```python
from build123d import *

# Parameters (mm, degrees)
BOSS_EXTRUDE9_DEPTH      = 12.7
SKETCH2_R                = 5.08
CUT_EXTRUDE1_DEPTH       = 1
CUT_EXTRUDE1_DEPTH_BACK  = 13.7
SKETCH4_R                = 5.08
CUT_EXTRUDE3_DEPTH       = 13.7
SKETCH6_W                = 63.5
SKETCH6_H                = 63.5
CUT_EXTRUDE10_DEPTH      = 8.382
SKETCH8_R                = 1.2954
CUT_EXTRUDE13_DEPTH      = 5.318
SKETCH20_R               = 1.045475937
SKETCH20_R_2             = 1.05
SKETCH20_R_3             = 1.053113333
SKETCH20_R_4             = 1.049702702
SKETCH20_R_5             = 1.060351353
SKETCH20_R_6             = 1.041366857
CUT_EXTRUDE14_DEPTH      = 5.318
SKETCH22_R               = 7.507138663
CUT_EXTRUDE15_DEPTH      = 12.742239248
SKETCH26_R               = 5.08
CUT_EXTRUDE16_DEPTH      = 1
CUT_EXTRUDE16_DEPTH_BACK = 13.7


with BuildPart() as part:
    # Sketch1 → Boss-Extrude9 (new body)
    with BuildSketch(Plane.XY):
        with BuildLine():
            Line((129.25673796, -48.023936093), (23.038420334, 135.95158673))
            ThreePointArc((23.038420334, 135.95158673), (0, 172.046968374), (-23.038420334, 135.95158673))
            Line((-23.038420334, 135.95158673), (-129.25673796, -48.023936093))
            ThreePointArc((-129.25673796, -48.023936093), (-148.997045256, -86.023484187), (-106.218317626, -87.927650637))
            Line((-106.218317626, -87.927650637), (106.218317626, -87.927650637))
            ThreePointArc((106.218317626, -87.927650637), (148.997045256, -86.023484187), (129.25673796, -48.023936093))
        make_face()
        with BuildLine():
            ThreePointArc((-121.92, -73.323484187), (-131.399409051, -75.863484187), (-124.46, -68.924075136))
            Line((-124.46, -68.924075136), (-127, -73.323484187))
            Line((-127, -73.323484187), (-121.92, -73.323484187))
        make_face(mode=Mode.SUBTRACT)
        with BuildLine():
            ThreePointArc((124.46, -68.924075136), (131.399409051, -75.863484187), (121.92, -73.323484187))
            Line((121.92, -73.323484187), (127, -73.323484187))
            Line((127, -73.323484187), (124.46, -68.924075136))
        make_face(mode=Mode.SUBTRACT)
        with BuildLine():
            ThreePointArc((-2.54, 142.247559323), (0, 151.726968374), (2.54, 142.247559323))
            Line((2.54, 142.247559323), (0, 146.646968374))
            Line((0, 146.646968374), (-2.54, 142.247559323))
        make_face(mode=Mode.SUBTRACT)
    extrude(amount=BOSS_EXTRUDE9_DEPTH)

    # Sketch2 → Cut-Extrude1 (cut, two sides)
    with BuildSketch(Plane.XY.offset(12.7)) as cut_extrude1_sk:
        with Locations((127, -73.323484187)):
            Circle(SKETCH2_R)
    extrude(amount=CUT_EXTRUDE1_DEPTH, mode=Mode.SUBTRACT)
    extrude(cut_extrude1_sk.sketch, amount=-CUT_EXTRUDE1_DEPTH_BACK, mode=Mode.SUBTRACT)

    # Sketch4 → Cut-Extrude3 (cut, through all)
    with BuildSketch(Plane.XY.offset(12.7)):
        with Locations((0, 146.646968374)):
            Circle(SKETCH4_R)
    extrude(amount=-CUT_EXTRUDE3_DEPTH, mode=Mode.SUBTRACT)

    # Sketch6 → Cut-Extrude10 (cut)
    with BuildSketch(Plane.XY.offset(12.7)):
        with Locations((0.191375803, -0.191375803)):
            Rectangle(SKETCH6_W, SKETCH6_H)
    extrude(amount=-CUT_EXTRUDE10_DEPTH, mode=Mode.SUBTRACT)

    # Sketch8 → Cut-Extrude13 (cut, through all)
    with BuildSketch(Plane.XY.offset(4.318)):
        with Locations((-25.511301342, -26.409321294)):
            Circle(SKETCH8_R)
        with Locations((-25.511301342, 26.803242123)):
            Circle(SKETCH8_R)
        with Locations((27.230878657, 26.803242123)):
            Circle(SKETCH8_R)
        with Locations((27.230878657, -26.409321294)):
            Circle(SKETCH8_R)
    extrude(amount=-CUT_EXTRUDE13_DEPTH, mode=Mode.SUBTRACT)

    # Sketch20 → Cut-Extrude14 (cut, through all)
    with BuildSketch(Plane.XY.offset(4.318)):
        with Locations((4.671117374, 6.592866865)):
            Circle(SKETCH20_R)
        with Locations((-2.048882626, 9.872866865)):
            Circle(SKETCH20_R_2)
        with Locations((-8.768882626, 6.592866865)):
            Circle(SKETCH20_R_3)
        with Locations((-12.048882626, -0.127133135)):
            Circle(SKETCH20_R_4)
        with Locations((-2.048882626, -10.127133135)):
            Circle(SKETCH20_R_5)
        with Locations((-8.768882626, -6.847133135)):
            Circle(SKETCH20_R_2)
        with Locations((4.671117374, -6.847133135)):
            Circle(SKETCH20_R_6)
    extrude(amount=-CUT_EXTRUDE14_DEPTH, mode=Mode.SUBTRACT)

    # Sketch22 → Cut-Extrude15 (cut, through all)
    with BuildSketch(Plane.XY.offset(11.742239248)):
        with Locations((-2.054203471, -0.131892244)):
            Circle(SKETCH22_R)
        with BuildLine():
            Line((3.541287317, -5.127133135), (7.21512242, -5.127133135))
            ThreePointArc((7.21512242, -5.127133135), (9.011173644, -4.38318436), (9.75512242, -2.587133135))
            Line((9.75512242, -2.587133135), (9.75512242, 2.341072368))
            ThreePointArc((9.75512242, 2.341072368), (9.011173644, 4.137123592), (7.21512242, 4.881072368))
            Line((7.21512242, 4.881072368), (3.541287317, 4.881072368))
            Line((3.541287317, 4.881072368), (3.541287317, -5.127133135))
        make_face()
    extrude(amount=-CUT_EXTRUDE15_DEPTH, mode=Mode.SUBTRACT)

    # Sketch26 → Cut-Extrude16 (cut, two sides)
    with BuildSketch(Plane.XY.offset(12.7)) as cut_extrude16_sk:
        with Locations((-127, -73.323484187)):
            Circle(SKETCH26_R)
    extrude(amount=CUT_EXTRUDE16_DEPTH, mode=Mode.SUBTRACT)
    extrude(cut_extrude16_sk.sketch, amount=-CUT_EXTRUDE16_DEPTH_BACK, mode=Mode.SUBTRACT)


solid = part.part
```
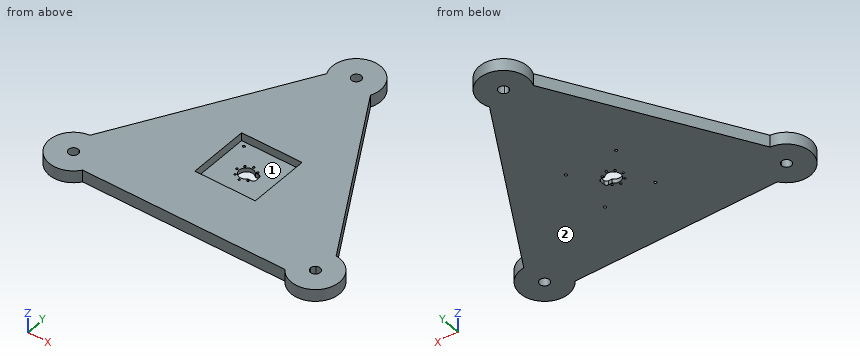
Design review of the part built by this model. Coordinates are the model's own, in mm. Face numbers are marked on the shaded views. Give positions to 0.01 mm unless a question says otherwise; leave off trailing zeros. Write each loop counter-clockwise with the first axis right and the second up, starting at its lowest first coordinate (ties: lowest second). Pieces come first, ordered by that corner, then holes.
(1) Wall thickness on line 1 along X through (y, z) = (146.5, 11.75); line 2 along X through (y, z) = (-76, 6.75); line 3 along Y through (x, z) = (-3, 9): over which ranges is each line inside the solid? List them lowest first.
Checked values:
line 1: x = -25.4 to -5.08, 5.08 to 25.4
line 2: x = -152.26 to -131.32, -122.68 to 122.68, 131.32 to 152.26
line 3: y = -87.93 to -31.94, 31.56 to 142.55, 150.75 to 171.87
(2) Clearance check with flat-ended pins moving along their axes: pin 1 Ø1.5 at (x, z) = (-43, 11.5) entering from -Y; pin 2 Ø6 at (y, z) = (114.5, 5.5) entering from +X; pin 3 Ø3.5 at (x, y) = (27.23, 26.8) entering from -Z; pin 4 Ø2.5 at (x, y) = (-2.05, 9.87) entering from +Z. State where each tip first meets the part, or that it passes through.
Checked values:
pin 1: stops at y = -87.93
pin 2: stops at x = 37.16
pin 3: stops at z = 0
pin 4: stops at z = 4.32
(3) Add section A-A (z = 7). Give the boundary of the cut face in (x, y), and give its area (3 significant figures).
Checked values:
outline: (-129.26, -48.02) arc R25.4 ccw (long way) to (-106.22, -87.93) - (106.22, -87.93) arc R25.4 ccw (long way) to (129.26, -48.02) - (23.04, 135.95) arc R25.4 ccw (long way) to (-23.04, 135.95) - close; hole circle Ø10.16 at (-127, -73.32); hole (-31.56, -31.94) - (31.94, -31.94) - (31.94, 31.56) - (-31.56, 31.56) - close; hole circle Ø10.16 at (0, 146.65); hole circle Ø10.16 at (127, -73.32)
area: 37,800 mm2
(4) Mouldability with a two-part tool opening along X and no side actions: class the marked faces 1 and 2 as +X half, -X half, draft (parallel to the pull), parting line (faces both ways), or undercut.
Checked values:
face 1: undercut
face 2: draft
(5) Add section C-C (x = 52). Give the boundary of the cut face in (y, z), and give its area (3 significant figures).
Checked values:
outline: (-87.93, 0) - (85.79, 0) - (85.79, 12.7) - (-87.93, 12.7) - close
area: 2,210 mm2
(6) Add section B-B (y = 16.5). Give the boundary of the cut face in (x, z).
Checked values:
outline: (-92, 0) - (92, 0) - (92, 12.7) - (31.94, 12.7) - (31.94, 4.32) - (-31.56, 4.32) - (-31.56, 12.7) - (-92, 12.7) - close
(7) Add section D-D (y = -61). Give the boundary of the cut face in (x, z), and give its area (3 significant figures).
Checked values:
outline: (-149.21, 0) - (149.21, 0) - (149.21, 12.7) - (-149.21, 12.7) - close
area: 3,790 mm2
